Build history of the part. All positions in model axes, mm. Coordinates: 2 decimals unless noted, no trailing zeros. Loops run counter-clockwise (first coordinate to the right, second up) from the corner with the lowest first, then second, coordinate; pieces in that order, holes last.
(1) Slice it at B-B (z = 95.5). Give the cut face in (x, y).
(2) Wall check: L1, parallel to Z at x = 91.5, y = 53; L2, parallel to X at y = 45, z = 273.5. Give the ranges that are in metal, low to high.
(3) Two-plate mould, pull along Z, no slides. Class faces 1 (the face through (328.412, 3, 349)), 2 (the face through (163, 3, 360)), 3 (the face through (11, -3, 1.588)): pulls with the +Z half, pulls with the -Z half, needs draft (parallel to the pull), parting line crosses it, or undercut.
(4) Flat gauge pins, fed straight in: P1, Ø1, axis at x = 176.5, y = -116, coming from the -Z side; P2, Ø12, axis at y = -138.5, z = 107, coming from the -X side; P3, Ø1.3, axis at y = 32.5, z = 0.5, coming from the +X side; P4, Ø0.5, axis at x = 329.5, y = 79.5, coming from the -Z side. Where does each tip first touch, or does it go through?
(5) Slice it at A-A (y = -41). Give the cut face in (x, z), and give its area (3 significant figures).
(6) Slice it at C-C (x = 304.5). Give the cut face in (y, z).
from build123d import *

# Parameters (mm, degrees)
SKETCH1_W                      = 1.5875
SKETCH1_H                      = 400
BASE_FLANGE1_DEPTH             = 360
EDGE_FLANGE1_STRIP_W           = 7.8232
EDGE_FLANGE1_STRIP_H           = 1.5875
EDGE_FLANGE1_STRIP_CUT_DEPTH   = 400
EDGE_FLANGE1_DEPTH             = 400
EDGE_FLANGE2_STRIP_W           = 7.8232
EDGE_FLANGE2_STRIP_H           = 1.5875
EDGE_FLANGE2_STRIP_CUT_DEPTH   = 400
EDGE_FLANGE2_STRIP_2_W         = 7.8232
EDGE_FLANGE2_STRIP_2_H         = 1.5875
EDGE_FLANGE2_STRIP_CUT_2_DEPTH = 400
EDGE_FLANGE2_DEPTH             = 400
EDGE_FLANGE2_BEND_DEPTH        = 400


# Sheet-metal steps are written as plain solids
with BuildPart() as part:
    # Sketch1 → Base-Flange1 (new body)
    with BuildSketch(Plane.XY):
        with Locations((0.79375, 0)):
            Rectangle(SKETCH1_W, SKETCH1_H)
    extrude(amount=BASE_FLANGE1_DEPTH)

    # Edge-Flange1 strip (across the edge) → Edge-Flange1 strip cut (cut)
    with BuildSketch(Plane(origin=(1.5875, 200, 360), x_dir=(0, 0, -1), z_dir=(0, -1, 0))):
        with Locations((-1.5875, -0.79375)):
            Rectangle(EDGE_FLANGE1_STRIP_W, EDGE_FLANGE1_STRIP_H)
    extrude(amount=EDGE_FLANGE1_STRIP_CUT_DEPTH, mode=Mode.SUBTRACT)

    # Edge-Flange1 section (across the edge) → Edge-Flange1 (add)
    with BuildSketch(Plane(origin=(1.5875, 200, 360), x_dir=(0, 0, -1), z_dir=(0, -1, 0))):
        with BuildLine():
            Line((0, 0.7366), (0, 328.4125))
            Line((0, 328.4125), (1.5875, 328.4125))
            Line((1.5875, 328.4125), (1.5875, 0.7366))
            ThreePointArc((1.5875, 0.7366), (1.803245145, 0.215745145), (2.3241, 0))
            Line((2.3241, 0), (2.3241, -1.5875))
            ThreePointArc((2.3241, -1.5875), (0.68071313, -0.90678687), (0, 0.7366))
        make_face()
    extrude(amount=EDGE_FLANGE1_DEPTH)

    # Edge-Flange2 strip (across the edge) → Edge-Flange2 strip cut (cut)
    with BuildSketch(Plane(origin=(330, 200, 358.4125), x_dir=(-1, 0, 0), z_dir=(0, -1, 0))):
        with Locations((-1.5875, -0.79375)):
            Rectangle(EDGE_FLANGE2_STRIP_W, EDGE_FLANGE2_STRIP_H)
    extrude(amount=EDGE_FLANGE2_STRIP_CUT_DEPTH, mode=Mode.SUBTRACT)

    # Edge-Flange2 strip 2 (across the edge) → Edge-Flange2 strip cut 2 (cut)
    with BuildSketch(Plane(origin=(1.5875, -200, 0), x_dir=(0, 0, 1), z_dir=(0, 1, 0))):
        with Locations((-1.5875, -0.79375)):
            Rectangle(EDGE_FLANGE2_STRIP_2_W, EDGE_FLANGE2_STRIP_2_H)
    extrude(amount=EDGE_FLANGE2_STRIP_CUT_2_DEPTH, mode=Mode.SUBTRACT)

    # Edge-Flange2 section (across the edge) → Edge-Flange2 (add)
    with BuildSketch(Plane(origin=(330, 200, 358.4125), x_dir=(-1, 0, 0), z_dir=(0, -1, 0))):
        with BuildLine():
            Line((0, 0.7366), (0, 18.4125))
            Line((0, 18.4125), (1.5875, 18.4125))
            Line((1.5875, 18.4125), (1.5875, 0.7366))
            ThreePointArc((1.5875, 0.7366), (1.803245145, 0.215745145), (2.3241, 0))
            Line((2.3241, 0), (2.3241, -1.5875))
            ThreePointArc((2.3241, -1.5875), (0.68071313, -0.90678687), (0, 0.7366))
        make_face()
    extrude(amount=EDGE_FLANGE2_DEPTH)

    # Edge-Flange2 section 2 (across the edge) → Edge-Flange2 bend (add)
    with BuildSketch(Plane(origin=(1.5875, -200, 0), x_dir=(0, 0, 1), z_dir=(0, 1, 0))):
        with BuildLine():
            Line((0, 0.7366), (0, 18.4125))
            Line((0, 18.4125), (1.5875, 18.4125))
            Line((1.5875, 18.4125), (1.5875, 0.7366))
            ThreePointArc((1.5875, 0.7366), (1.803245145, 0.215745145), (2.3241, 0))
            Line((2.3241, 0), (2.3241, -1.5875))
            ThreePointArc((2.3241, -1.5875), (0.68071313, -0.90678687), (0, 0.7366))
        make_face()
    extrude(amount=EDGE_FLANGE2_BEND_DEPTH)


solid = part.part
Response values:
1. outline: (0, -200) - (1.59, -200) - (1.59, 200) - (0, 200) - close
2. L1: z = 358.41 to 360
2. L2: x = 0 to 1.59
3. face 1: needs draft
3. face 2: pulls with the +Z half
3. face 3: undercut
4. P1: stops at z = 358.41
4. P2: stops at x = 0
4. P3: stops at x = 20
4. P4: stops at z = 340
5. outline: (0, 2.32) arc R2.32 ccw to (2.32, 0) - (20, 0) - (20, 1.59) - (2.32, 1.59) arc R0.74 cw to (1.59, 2.32) - (1.59, 357.68) arc R0.74 cw to (2.32, 358.41) - (327.68, 358.41) arc R0.74 cw to (328.41, 357.68) - (328.41, 340) - (330, 340) - (330, 357.68) arc R2.32 ccw to (327.68, 360) - (2.32, 360) arc R2.32 ccw to (0, 357.68) - close
5. area: 1,150 mm2
6. outline: (-200, 358.41) - (200, 358.41) - (200, 360) - (-200, 360) - close
